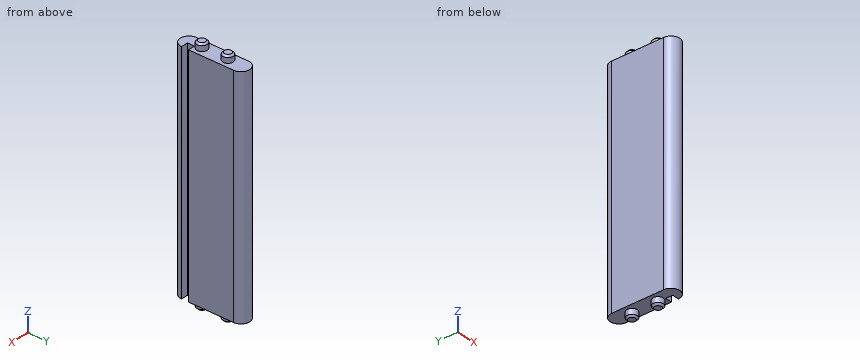
```python
from build123d import *

# Parameters (mm, degrees)
EXTRUDE_1_DEPTH            = 65
SKETCH_2_R                 = 3
EXTRUDE_2_DEPTH            = 4
CHAMFER_1_SIZE             = 1
CHAMFER_1_OF_MIRROR_1_SIZE = 1


with BuildPart() as part:
    # 草圖1 → 伸長1 (new, symmetric)
    with BuildSketch(Plane.XY):
        with BuildLine():
            Line((-5, 15), (-5, -15))
            ThreePointArc((-5, -15), (0, -20), (5, -15))
            Line((5, -15), (1, -15))
            Line((1, -15), (1, -11))
            Line((1, -11), (5, -11))
            Line((5, -11), (5, 15))
            ThreePointArc((5, 15), (0, 20), (-5, 15))
        make_face()
    extrude(amount=EXTRUDE_1_DEPTH, both=True)

    # 草圖2 → 伸長2 (add)
    with BuildSketch(Plane.XY.offset(65)):
        with Locations(Location((0, 7.5, 0), (0, 0, 180))):
            Circle(SKETCH_2_R)
        with Locations(Location((0, -7.5, 0), (0, 0, 180))):
            Circle(SKETCH_2_R)
    extrude_2 = extrude(amount=EXTRUDE_2_DEPTH)

    # 導角1
    chamfer_1_edges = [part.edges().sort_by_distance(p)[0] for p in [
        (3, 7.5, 69),
        (3, -7.5, 69),
    ]]
    chamfer(chamfer_1_edges, length=CHAMFER_1_SIZE)

    # 鏡射1: 伸長2 across plane
    add(extrude_2.mirror(Plane.XY))

    # 導角1 of 鏡射1
    chamfer_1_of_mirror_1_edges = [part.edges().sort_by_distance(p)[0] for p in [
        (3, 7.5, -69),
        (3, -7.5, -69),
    ]]
    chamfer(chamfer_1_of_mirror_1_edges, length=CHAMFER_1_OF_MIRROR_1_SIZE)


solid = part.part
```
The listing builds one solid part. Answer for the finished solid, in the listing's coordinates (mm). Give positions to 0.01 mm unless a question says otherwise; leave off trailing zeros. Order: outer loops, then holes, each group sorted by start corner. A loop starts at its lowest first (then second) coordinate and runs counter-clockwise, first axis right, second up. Notation, with made-up numbers: (63, 46) -> (72, 46) arc R23 cw to (72, 69) -> close; hole circle Ø8 at (36, 1). An arc over 180 degrees is marked (long way). One line per item, written item: value.
1) Find section A-A, the plane y = -7.5. Determine the outline of the cut face in (x, z).
Reported:
outline: (-5, -65) -> (-3, -65) -> (-3, -68) -> (-2, -69) -> (2, -69) -> (3, -68) -> (3, -65) -> (5, -65) -> (5, 65) -> (3, 65) -> (3, 68) -> (2, 69) -> (-2, 69) -> (-3, 68) -> (-3, 65) -> (-5, 65) -> close
2) Find section D-D, the plane y = 13.5. Determine the outline of the cut face in (x, z), plus the area to 3 significant figures.
Reported:
outline: (-5, -65) -> (5, -65) -> (5, 65) -> (-5, 65) -> close
area: 1,300 mm^2
3) Flat-ended cylindrical pins translate along their axes: P1, Ø2, axis at x = 3.5, z = -16.5, coming from the -Y side; P2, Ø2, axis at x = 2.5, z = 2, coming from the +Y side; P3, Ø3, axis at x = -2.5, y = -2.5, coming from the +Z side. Find the tip coordinate at first contact, or state that the pin passes through.
Reported:
P1: stops at y = -19.33
P2: stops at y = 19.77
P3: stops at z = 65
4) Find section C-C, the plane y = -18. Determine the outline of the cut face in (x, z), plus the area to 3 significant figures.
Reported:
outline: (-4, -65) -> (4, -65) -> (4, 65) -> (-4, 65) -> close
area: 1,040 mm^2
5) Find the intervals of material crossed by line 1 (Z direction, x = 1, y = -17); line 2 (X direction, y = -12.5, z = -47.5); line 3 (Y direction, x = 3.5, z = -0.5), in increasing order.
Reported:
line 1: z = -65 to 65
line 2: x = -5 to 1
line 3: y = -18.57 to -15, -11 to 18.57
6) Find section B-B, the plane z = 11. Determine the outline of the cut face in (x, y), plus the area to 3 significant figures.
Reported:
outline: (-5, -15) arc R5 ccw to (5, -15) -> (1, -15) -> (1, -11) -> (5, -11) -> (5, 15) arc R5 ccw to (-5, 15) -> close
area: 363 mm^2
